from build123d import *

# Parameters (mm, degrees)
F0_W     = 152.4
F0_H     = 152.4
F1_DEPTH = 762
F3_DEPTH = 152.4
F5_DEPTH = 152.4


with BuildPart() as f1:
    # F0 (on Right) → F1 (new body)
    with BuildSketch(Plane.YZ):
        Rectangle(F0_W, F0_H)
    extrude(amount=F1_DEPTH)

    # F2 (on face) → F3 (cut)
    with BuildSketch(Plane.XY.offset(76.2)):
        Polygon((762, -12.7), (152.4, -76.2), (762, -76.2), align=None)
    extrude(amount=-F3_DEPTH, mode=Mode.SUBTRACT)

    # F4 (on face) → F5 (cut)
    with BuildSketch(Plane(origin=(0, 76.2, 0), x_dir=(-1, 0, 0), z_dir=(0, 1, 0))):
        Polygon((-762, 12.7), (-152.4, 76.2), (-762, 76.2), align=None)
    extrude(amount=-F5_DEPTH, mode=Mode.SUBTRACT)


solid = f1.part
Part model, mm, in its own coordinate system. Give positions to 0.01 mm unless a question says otherwise; leave off trailing zeros. Order: outer loops, then holes, each group sorted by start corner. A loop starts at its lowest first (then second) coordinate and runs counter-clockwise, first axis right, second up. Notation, with made-up numbers: (65, 58) - (123, 58) arc R18 cw to (123, 70) - close; hole circle Ø11 at (34.5, 54). An arc over 180 degrees is marked (long way). Use a Markdown table: item, result.
1) Saw through at B-B on y = -37. List the corners of the cut face in (x, z), plus the area to 3 significant figures.
Checked values:
| item | result |
|---|---|
| outline | (0, -76.2) - (528.72, -76.2) - (528.72, 37) - (152.4, 76.2) - (0, 76.2) - close |
| area | 73,200 mm² |
2) Saw through at C-C on x = 618. List the corners of the cut face in (y, z), plus the area to 3 significant figures.
Checked values:
| item | result |
|---|---|
| outline | (-27.7, -76.2) - (76.2, -76.2) - (76.2, 27.7) - (-27.7, 27.7) - close |
| area | 10,800 mm² |
3) Probe L1, parallel to Z at x = 315.5, y = 45; L2, parallel to Y at x = 620.5, z = 15.5; L3, parallel to Y at x = 542, z = -59. List the from-to ranges inside material, lowest first. Write a range as from..to.
Checked values:
| item | result |
|---|---|
| L1 | -76.2..59.21 |
| L2 | -27.44..76.2 |
| L3 | -35.62..76.2 |
4) Flat gauge pins, fed straight in: P1, Ø4, axis at x = 379, y = -23, coming from the +Z side; P2, Ø10, axis at x = 250.5, y = 21, coming from the +Z side; P3, Ø12, axis at x = 245.5, z = -21, coming from the -Y side. Where does each tip first touch, or does it go through?
Checked values:
| item | result |
|---|---|
| P1 | z = 52.8 |
| P2 | z = 66.5 |
| P3 | y = -67.13 |
5) Saw through at A-A on z = 48.5. List the corners of the cut face in (x, y), plus the area to 3 significant figures.
Checked values:
| item | result |
|---|---|
| outline | (0, -76.2) - (152.4, -76.2) - (418.32, -48.5) - (418.32, 76.2) - (0, 76.2) - close |
| area | 60,100 mm² |
6) Saw through at D-D on x = 329.5. List the corners of the cut face in (y, z), plus the area to 3 significant figures.
Checked values:
| item | result |
|---|---|
| outline | (-57.75, -76.2) - (76.2, -76.2) - (76.2, 57.75) - (-57.75, 57.75) - close |
| area | 17,900 mm² |
